Read the model definition and answer for the solid it produces. Units are mm, in the model's axes. A direction names the side the tool comes from. Round coordinates to 2 decimals unless told otherwise and drop trailing zeros. Write each loop counter-clockwise with the first axis right and the second up, starting at its lowest first coordinate (ties: lowest second). Pieces come first, ordered by that corner, then holes. Notation, with made-up numbers: (72.5, 47.5) - (78.5, 47.5) arc R24 ccw to (78.5, 71.5) - close; hole circle Ø10 at (-21.5, 49). An arc over 180 degrees is marked (long way). Use one line per item in the form item = value. Start each with the question number.
1) The part is cut by section D-D, the plane z = 1.5. Give the vertices of the cut face in (x, y), plus the area to 3 significant figures.
2) The part is cut by section C-C, the plane y = 0. Give the vertices of the cut face in (x, z).
3) The part is cut by section A-A, the plane x = 142. Give the vertices of the cut face in (y, z), plus the area to 3 significant figures.
4) Consider line 1 along Y through (x, z) = (165, 2.5); line 2 along Y through (x, z) = (164.25, 5.1); line 3 along X through (y, z) = (-0.25, 7.75). Determine where each line is inside the solid, lowest interval first. Write a range as from..to.
5) The part is cut by section B-B, the plane y = 4.75. Give the vertices of the cut face in (x, z).
6) Each of these flat-tipped pins is pushed along its axis until it touches: pin 1 (5 mm diameter, centred on x = 137, y = 1, fed in from +Z); pin 2 (2 mm diameter, centred on x = 165, y = -1.5, fed in from -Z); pin 3 (3.5 mm diameter, centred on x = 165.5, y = 2, fed in from +Z). Where does it stop, or does it pass through?
7) For faces 1 (the face through (150, -7.494, 5)), 2 (the face through (133.519, 0, 8)), 3 (the face through (166.919, 0, 2)), 4 (the face through (132.363, 0, 5)), 5 (the face through (162.419, 0, 5)), determine the directions among +Z, -Z, +X, -X, +Y, -Y from which every point of the face is accessible in a straight line to the end or side of a thin tool.
from build123d import *

# Parameters (mm, degrees)
BOSS_EXTRUDE1_DEPTH = 25
SKETCH16_W          = 33.4
SKETCH16_H          = 13.3
CUT_EXTRUDE10_DEPTH = 4.5
SKETCH19_R          = 20
CUT_EXTRUDE14_DEPTH = 5
SKETCH17_W          = 24.4
SKETCH17_H          = 13.3
CUT_EXTRUDE11_DEPTH = 177.45821035
CUT_EXTRUDE13_DEPTH = 6.45
SKETCH20_W          = 33.4
SKETCH20_H          = 13.3
CUT_EXTRUDE15_DEPTH = 176.655202029
SKETCH21_R          = 1.1
CUT_EXTRUDE16_DEPTH = 177.45821035
SKETCH22_R          = 2
CUT_EXTRUDE17_DEPTH = 20
SKETCH23_W          = 35.542805721
SKETCH23_H          = 15.334329657
SKETCH23_R          = 20
CUT_EXTRUDE18_DEPTH = 177.45821035
SKETCH24_W          = 18.060519465
SKETCH24_H          = 23.66068054
CUT_EXTRUDE19_DEPTH = 45.156146987


with BuildPart() as part:
    # Sketch1 → Boss-Extrude1 (new body)
    with BuildSketch(Plane.XY):
        with BuildLine():
            ThreePointArc((172.5, 0), (152.823244805, 26.363741023), (121.951138857, 15))
            Line((121.951138857, 15), (145, 15))
            Line((145, 15), (145, -15))
            Line((145, -15), (121.951138857, -15))
            ThreePointArc((121.951138857, -15), (152.823244805, -26.363741023), (172.5, 0))
        make_face()
        with BuildLine():
            Line((145, 15), (121.951138857, 15))
            ThreePointArc((121.951138857, 15), (117.5, 0), (121.951138857, -15))
            Line((121.951138857, -15), (145, -15))
            Line((145, -15), (145, 15))
        make_face()
        with BuildLine():
            Line((121.951138857, 15), (23.048861143, 15))
            ThreePointArc((23.048861143, 15), (26.363741023, 7.823244805), (27.5, 0))
            ThreePointArc((27.5, 0), (26.363741023, -7.823244805), (23.048861143, -15))
            Line((23.048861143, -15), (121.951138857, -15))
            ThreePointArc((121.951138857, -15), (117.5, 0), (121.951138857, 15))
        make_face()
        with BuildLine():
            ThreePointArc((13.228756555, -15), (-20, 0), (13.228756555, 15))
            Line((13.228756555, 15), (23.048861143, 15))
            ThreePointArc((23.048861143, 15), (-27.5, 0), (23.048861143, -15))
            Line((23.048861143, -15), (13.228756555, -15))
        make_face()
        with BuildLine():
            Line((23.048861143, 15), (13.228756555, 15))
            ThreePointArc((13.228756555, 15), (18.228756555, 8.228756555), (20, 0))
            ThreePointArc((20, 0), (18.228756555, -8.228756555), (13.228756555, -15))
            Line((13.228756555, -15), (23.048861143, -15))
            ThreePointArc((23.048861143, -15), (26.363741023, -7.823244805), (27.5, 0))
            ThreePointArc((27.5, 0), (26.363741023, 7.823244805), (23.048861143, 15))
        make_face()
        with BuildLine():
            Line((0, -15), (0, 15))
            Line((0, 15), (13.228756555, 15))
            ThreePointArc((13.228756555, 15), (-20, 0), (13.228756555, -15))
            Line((13.228756555, -15), (0, -15))
        make_face()
        with BuildLine():
            Line((13.228756555, 15), (0, 15))
            Line((0, 15), (0, -15))
            Line((0, -15), (13.228756555, -15))
            ThreePointArc((13.228756555, -15), (18.228756555, -8.228756555), (20, 0))
            ThreePointArc((20, 0), (18.228756555, 8.228756555), (13.228756555, 15))
        make_face()
    extrude(amount=BOSS_EXTRUDE1_DEPTH)

    # Sketch16 → Cut-Extrude10 (cut)
    with BuildSketch(Plane(origin=(0, 0, 0), x_dir=(-1, 0, 0), z_dir=(0, 0, -1))):
        with Locations((-150.21934279, 0)):
            Rectangle(SKETCH16_W, SKETCH16_H)
    extrude(amount=-CUT_EXTRUDE10_DEPTH, mode=Mode.SUBTRACT)

    # Sketch19 → Cut-Extrude14 (cut)
    with BuildSketch(Plane(origin=(0, 0, 0), x_dir=(-1, 0, 0), z_dir=(0, 0, -1))):
        Circle(SKETCH19_R)
    extrude(amount=-CUT_EXTRUDE14_DEPTH, mode=Mode.SUBTRACT)

    # Sketch17 → Cut-Extrude11 (cut, through all)
    with BuildSketch(Plane(origin=(0, 0, 0), x_dir=(-1, 0, 0), z_dir=(0, 0, -1))):
        with Locations((-150.21934279, 0)):
            Rectangle(SKETCH17_W, SKETCH17_H)
    extrude(amount=-CUT_EXTRUDE11_DEPTH, mode=Mode.SUBTRACT)

    # Sketch18 → Cut-Extrude13 (cut, symmetric)
    with BuildSketch(Plane(origin=(0, 0, 0), x_dir=(-1, 0, 0), z_dir=(0, -1, 0))):
        Polygon((-138.01934279, -15), (-138.01934279, -25), (-122.01934279, -25), (-122.01934279, -22.5), align=None)
    extrude(amount=CUT_EXTRUDE13_DEPTH, both=True, mode=Mode.SUBTRACT)

    # Sketch20 → Cut-Extrude15 (cut, through all)
    with BuildSketch(Plane(origin=(0, 0, 6.5), x_dir=(-1, 0, 0), z_dir=(0, 0, -1))):
        with Locations((-150.21934279, 0)):
            Rectangle(SKETCH20_W, SKETCH20_H)
    extrude(amount=-CUT_EXTRUDE15_DEPTH, mode=Mode.SUBTRACT)

    # Sketch21 → Cut-Extrude16 (cut, through all)
    with BuildSketch(Plane(origin=(0, 0, 0), x_dir=(-1, 0, 0), z_dir=(0, 0, -1))):
        with Locations((-164.249999957, 0)):
            Circle(SKETCH21_R)
        with Locations((-136.249999957, 0)):
            Circle(SKETCH21_R)
    extrude(amount=-CUT_EXTRUDE16_DEPTH, mode=Mode.SUBTRACT)

    # Sketch22 → Cut-Extrude17 (cut)
    with BuildSketch(Plane.XY.offset(25)):
        Circle(SKETCH22_R)
    extrude(amount=-CUT_EXTRUDE17_DEPTH, mode=Mode.SUBTRACT)

    # Sketch23 → Cut-Extrude18 (cut, through all)
    with BuildSketch(Plane(origin=(0, 0, 0), x_dir=(-1, 0, 0), z_dir=(0, 0, -1))):
        with BuildLine():
            ThreePointArc((-121.951138857, 15), (-172.5, 0), (-121.951138857, -15))
            Line((-121.951138857, -15), (-23.048861143, -15))
            ThreePointArc((-23.048861143, -15), (27.5, 0), (-23.048861143, 15))
            Line((-23.048861143, 15), (-121.951138857, 15))
        make_face()
        with Locations((-150.134671958, 0.173388614)):
            Rectangle(SKETCH23_W, SKETCH23_H, mode=Mode.SUBTRACT)
        Circle(SKETCH23_R, mode=Mode.SUBTRACT)
    extrude(amount=-CUT_EXTRUDE18_DEPTH, mode=Mode.SUBTRACT)


with BuildPart() as cut_extrude18_kept_piece:
    # of the separate pieces the step leaves, the one the design keeps (cut_extrude18_pieces_kept)
    add(part.part.solids().sort_by_distance((133.51934279, 6.45, 25))[0])

    # Sketch24 → Cut-Extrude19 (cut, through all)
    with BuildSketch(Plane.ZY.offset(-132.363269097)):
        with Locations((18.423868143, -1.593012334)):
            Rectangle(SKETCH24_W, SKETCH24_H)
    extrude(amount=-CUT_EXTRUDE19_DEPTH, mode=Mode.SUBTRACT)


solid = cut_extrude18_kept_piece.part
Geometry results:
q1.outline = (132.36, -7.49) - (167.91, -7.49) - (167.91, 7.84) - (132.36, 7.84) - close; hole (133.52, -6.65) - (166.92, -6.65) - (166.92, 6.65) - (133.52, 6.65) - close
q1.area = 101 mm2
q2.outline = (132.36, 0) - (133.52, 0) - (133.52, 4.5) - (135.15, 4.5) - (135.15, 6.5) - (133.52, 6.5) - (133.52, 9.39) - (132.36, 9.39) - close; (137.35, 4.5) - (138.02, 4.5) - (138.02, 6.5) - (137.35, 6.5) - close; (162.42, 4.5) - (163.15, 4.5) - (163.15, 6.5) - (162.42, 6.5) - close; (165.35, 4.5) - (166.92, 4.5) - (166.92, 0) - (167.91, 0) - (167.91, 9.39) - (166.92, 9.39) - (166.92, 6.5) - (165.35, 6.5) - close
q3.outline = (-7.49, 0) - (-6.65, 0) - (-6.65, 9.39) - (-7.49, 9.39) - close; (6.65, 0) - (7.84, 0) - (7.84, 9.39) - (6.65, 9.39) - close
q3.area = 19.1 mm2
q4.line_1 = -7.49..-6.65, 6.65..7.84
q4.line_2 = -7.49..-1.1, 1.1..7.84
q4.line_3 = 132.36..133.52, 166.92..167.91
q5.outline = (132.36, 0) - (133.52, 0) - (133.52, 4.5) - (138.02, 4.5) - (138.02, 6.5) - (133.52, 6.5) - (133.52, 9.39) - (132.36, 9.39) - close; (162.42, 4.5) - (166.92, 4.5) - (166.92, 0) - (167.91, 0) - (167.91, 9.39) - (166.92, 9.39) - (166.92, 6.5) - (162.42, 6.5) - close
q6.pin_1 = 6.5
q6.pin_2 = 4.5
q6.pin_3 = 9.39
q7.face_1 = +Z, -Z, +X, -X, -Y
q7.face_2 = +Z
q7.face_3 = -Z
q7.face_4 = +Z, -Z, -X, +Y, -Y
q7.face_5 = +Z, -Z
